Autodesk Inventor part; units mm, degrees
ref_plane "YZ Plane" through (0, 0, 0) normal (1, 0, 0) x (0, 1, 0)
ref_plane "XZ Plane" through (0, 0, 0) normal (0, 1, 0) x (-1, 0, 0)
ref_plane "XY Plane" through (0, 0, 0) normal (0, 0, 1) x (1, 0, 0)
sketch "Sketch1" plane through (0, 0, 0) normal (0, 1, 0) x (-1, 0, 0)
  line L0 (-54, 0) -> (-54, -86)
  line L1 (-54, -86) -> (0, -86)
  line L2 (0, -86) -> (0, 0)
  line L3 (0, 0) -> (-2, 0) construction
  line L4 (-2, 0) -> (-2, -4) construction
  line L5 (0, -86) -> (0, -84) construction
  line L6 (-52, -4) -> (-52, -84)
  line L7 (-52, -84) -> (-2, -84)
  line L8 (-2, -84) -> (-2, -4)
  line L9 (-25, 0) -> (-25, -4)
  line L10 (-29, 0) -> (-29, -4)
  line L11 (-2, -4) -> (-25, -4)
  line L12 (-29, -4) -> (-52, -4)
  line L13 (0, 0) -> (-25, 0)
  line L14 (-29, 0) -> (-54, 0)
  point P0 (-25, -2)
  dimension "d1" = 54
  dimension "d2" = 86
  dimension "d3" = 2
  dimension "d4" = 4
  dimension "d5" = 2
  dimension "d6" = 50
  dimension "d7" = 25
  dimension "d8" = 29
extrude "Extrusion1" add sketch "Sketch1" along normal blind 2
ref_plane "Work Plane1" through (0, 2, 0) normal (0, 0.9999, -0.0118) x (1, 0, 0)
sketch "Sketch2" plane through (0, 2, 0) normal (0, 0.9999, -0.0118) x (1, 0, 0)
  line L0 (-35.8906, -24.3728) -> (94.8707, -24.3728)
  line L1 (94.8707, -24.3728) -> (94.8707, 112.0739)
  line L2 (94.8707, 112.0739) -> (-35.8906, 112.0739)
  line L3 (-35.8906, 112.0739) -> (-35.8906, -24.3728)
  point P0 (0, 0.0236)
extrude "Extrusion2" cut sketch "Sketch2" along normal blind 8.25
properties part number "wing0.3.1_conductive"
Geometry check sheet. Reference: the model listing, model coordinates, mm. A direction names the side the tool comes from. Round coordinates to 2 decimals unless told otherwise and drop trailing zeros. Order: outer loops, then holes, each group sorted by start corner. A loop starts at its lowest first (then second) coordinate and runs counter-clockwise, first axis right, second up. Notation, with made-up numbers: M -8.5,63 L 30.5,63 A18 cw 30.5,87 Z; hole C 0.25,-4 d6. An arc over 180 degrees is marked long. Answer in a Markdown table with one row per item. Add a question column.
Item 1: Set-up check for faces 1 (the face through (25, 1, -2)), 2 (the face through (12, 1, 0)), 3 (the face through (13, 1, -4)): record each of +Z, -Z, +X, -X, +Y, -Y from which the full face is reachable in a straight line by a thin tool's end or side.
Item 2: Sectioned sample at B-B, the plane z = -59.5. Enter the section's corners in (x, y).
Item 3: Material ranges on L1, parallel to X at y = 1.6, z = -30; L2, parallel to Z at x = 3, y = 0.95; L3, parallel to Z at x = 48, y = 1.05, recorded low to high. Write a range as [from, to].
Item 4: Sectioned sample at A-A, the plane x = 33. Enter the section's corners in (y, z), plus the area to 3 significant figures.
Item 5: Sectioned sample at C-C, the plane y = 0.4. Enter the section's corners in (x, z), plus the area to 3 significant figures.
Item 6: Depth check by flat-ended pin: pin 1 Ø0.5 at (x, y) = (26, 0.5) entering from +Z; pin 2 Ø12 at (x, z) = (40, -9) entering from +Y. Enter the tip coordinate at first touch or a pass-through.
Item 7: Draft check along X on faces 4 (the face through (54, 1, -42)), 5 (the face through (41, 1, 0)), 6 (the face through (2, 1, -45)). Enter one of: released by +X, released by -X, zero draft, split by the parting line, or undercut.
Filled in:
| question | item | result |
|---|---|---|
| 1 | face 1 | +Z, +Y, -Y |
| 1 | face 2 | +Z, +X, -X, +Y, -Y |
| 1 | face 3 | +Y, -Y |
| 2 | outline | M 0,0 L 2,0 L 2,1.3 L 0,1.3 Z; M 52,0 L 54,0 L 54,1.3 L 52,1.3 Z |
| 3 | L1 | x = [0, 2], [52, 54] |
| 3 | L2 | z = [-86, -84], [-4, 0] |
| 3 | L3 | z = [-4, 0] |
| 4 | outline | M 0,-86 L 0.98,-86 L 1.01,-84 L 0,-84 Z; M 0,-4 L 1.95,-4 L 2,0 L 0,0 Z |
| 4 | area | 9.89 mm² |
| 5 | outline | M 0,-86 L 54,-86 L 54,0 L 29,0 L 29,-4 L 52,-4 L 52,-84 L 2,-84 L 2,-4 L 25,-4 L 25,0 L 0,0 Z |
| 5 | area | 628 mm² |
| 6 | pin 1 | stops at z = -84 |
| 6 | pin 2 | stops at y = 1.96 |
| 7 | face 4 | released by +X |
| 7 | face 5 | zero draft |
| 7 | face 6 | undercut |
